Input: part model. Units: mm. Frame: model coordinates. Face numbers are marked on the shaded views. A direction names the side the tool comes from. Coordinates: 2 decimals unless noted, no trailing zeros. Order: outer loops, then holes, each group sorted by start corner. A loop starts at its lowest first (then second) coordinate and runs counter-clockwise, first axis right, second up.
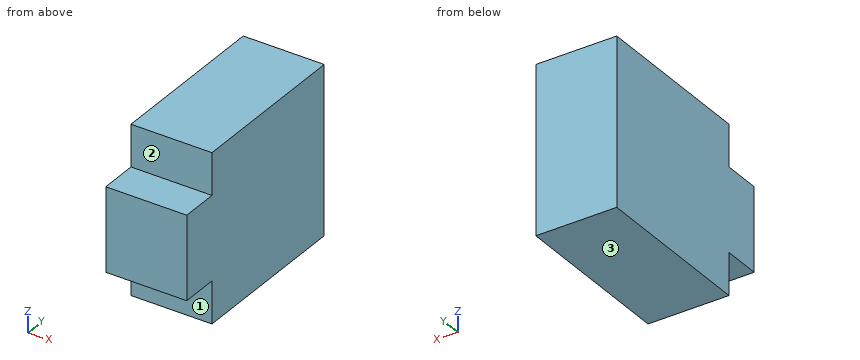
Autodesk Inventor part; units mm, degrees
ref_plane "YZ Plane" through (0, 0, 0) normal (1, 0, 0) x (0, 1, 0)
ref_plane "XZ Plane" through (0, 0, 0) normal (0, 1, 0) x (-1, 0, 0)
ref_plane "XY Plane" through (0, 0, 0) normal (0, 0, 1) x (1, 0, 0)
sketch "Sketch1" plane through (0, 0, 0) normal (0, 1, 0) x (-1, 0, 0)
  line L0 (4.3357, 14.1429) -> (-12.2143, 14.1429)
  line L1 (-12.2143, 14.1429) -> (-12.2143, -20.0571)
  line L2 (-12.2143, -20.0571) -> (4.3357, -20.0571)
  line L3 (4.3357, -20.0571) -> (4.3357, 14.1429)
  point P0 (0, 0)
  dimension "d0" = 34.2
  dimension "d1" = 16.55
extrude "Extrusion1" add sketch "Sketch1" along normal blind 42
sketch "Sketch2" plane through (12.2143, 0, 14.1429) normal (1, 0, 0) x (0, 0, -1)
  circle A0 centre (17.1, 24.85) radius 1.9655
  line L0 (0, 42) -> (34.2, 42)
  line L1 (0, 0) -> (0, 42)
  point P0 (14.1429, 0)
  dimension "d4" = 17.15
  dimension "d5" = 17.1
sketch "Sketch3" plane through (12.2143, 0, 14.1429) normal (1, 0, 0) x (0, 0, -1)
  line L0 (0, 0) -> (8.53, 0)
  line L1 (8.53, 0) -> (8.53, 7.7)
  line L2 (8.53, 7.7) -> (0, 7.7)
  line L3 (0, 7.7) -> (0, 0)
  point P0 (14.1429, 0)
  dimension "d18" = 7.7
  dimension "d19" = 8.53
extrude "Extrusion2" cut sketch "Sketch3" against normal blind 17.9375
sketch "Sketch4" plane through (12.2143, 0, -20.0571) normal (1, 0, 0) x (0, 0, -1)
  line L0 (0, 0) -> (0, 42)
  line L1 (0, 0) -> (-8.6, 0)
  line L2 (-8.6, 0) -> (-8.6, 7.7)
  line L3 (-8.6, 7.7) -> (0, 7.7)
  line L4 (0, 7.7) -> (0, 0)
  point P0 (-20.0571, 0)
  point P1 (0, 7.7)
  dimension "d22" = 8.6
  dimension "d23" = 7.7
extrude "Extrusion3" cut sketch "Sketch4" against normal blind 17.9375
properties part number "Arducam_Mega"
Item 1: Ray query, probe 1 along Y at (x, z) = (6, -16); probe 2 along Z at (x, y) = (5.75, 4). Return the intervals inside material, ascending.
Response values:
probe 1: y = 7.7 to 42
probe 2: z = -11.46 to 5.61
Item 2: Access query for the marked faces 1, 2 and 3. Directions: +Z, -Z, +X, -X, +Y, -Y. A direction counts if a zero-diameter tool reaches every point of the face in a straight line with its end or side. Return the directions, or none.
Response values:
face 1: -Z, +X, -X, -Y
face 2: +Z, +X, -X, -Y
face 3: -Z, +X, -X, +Y, -Y
Item 3: Cut plane B-B on z = -13.5. Return loops of the section in (x, y).
Response values:
outline: (-4.34, 7.7) - (12.21, 7.7) - (12.21, 42) - (-4.34, 42) - close
Item 4: Pin query (flat end, axial travel): pin 1 Ø8.5 at (x, y) = (6.5, 3.5) entering from -Z; pin 2 Ø2.5 at (x, y) = (0, 4.5) entering from +Z; pin 3 Ø4.5 at (x, z) = (0.5, 10.5) entering from -Y. Return the tip coordinate at first contact, or that it passes through.
Response values:
pin 1: stops at z = -20.06
pin 2: stops at z = 5.61
pin 3: stops at y = 7.7
Item 5: Cut plane A-A on x = 2.25. Return loops of the section in (y, z).
Response values:
outline: (0, -11.46) - (7.7, -11.46) - (7.7, -20.06) - (42, -20.06) - (42, 14.14) - (7.7, 14.14) - (7.7, 5.61) - (0, 5.61) - close
